The figure shows three views and two pictorial views of one solid part (mm, origin at its lowest corner). Answer the questions. Give positions to 0.01 mm unless a question says otherwise; leave off trailing zeros. Loops run counter-clockwise (first coordinate to the right, second up) from the corner with the lowest first, then second, coordinate; pieces in that order, holes last. Notation, with made-up numbers: (20, -30) - (77, -30) arc R37 ccw to (77, 7) - close; hole circle Ø5 at (26.5, 7.5). An arc over 180 degrees is marked (long way). One line per question, with ' | ' between items.
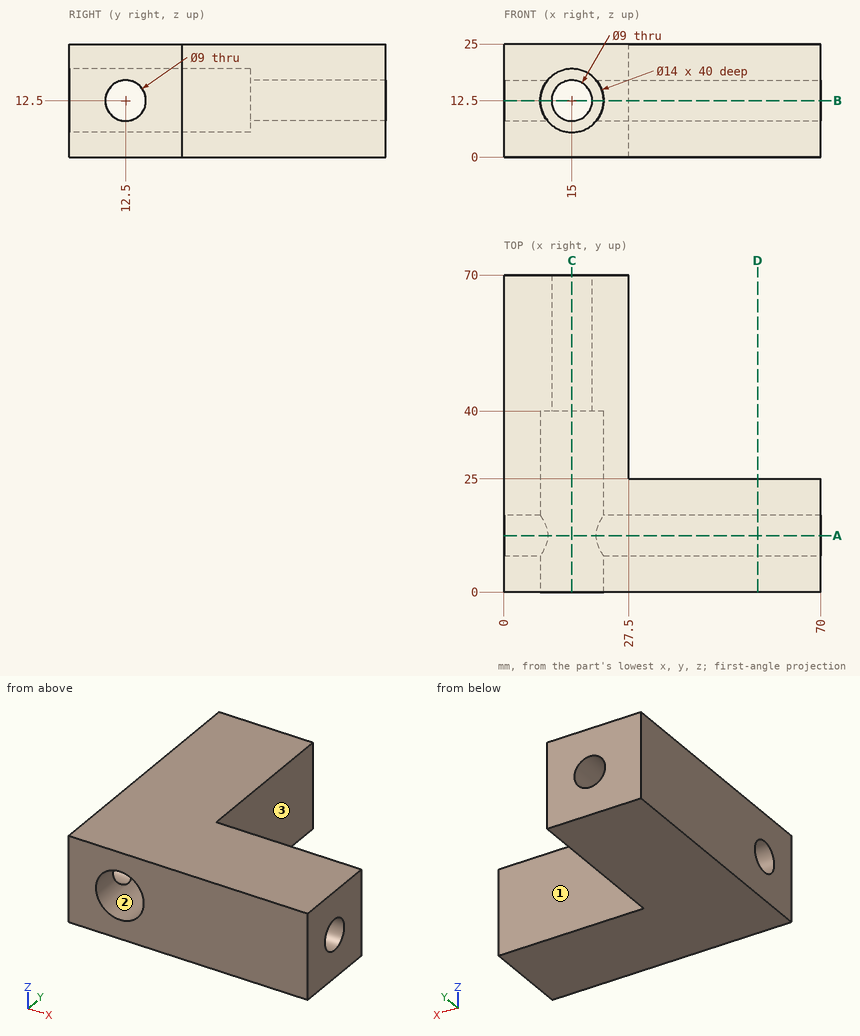
1. Find section B-B on z = 12.5. Write down the section's boundary in (x, y).
Evaluation:
outline: (0, 0) - (8, 0) - (8, 8) - (0, 8) - close; (0, 17) - (8, 17) - (8, 40) - (10.5, 40) - (10.5, 70) - (0, 70) - close; (19.5, 40) - (22, 40) - (22, 17) - (70, 17) - (70, 25) - (27.5, 25) - (27.5, 70) - (19.5, 70) - close; (22, 0) - (70, 0) - (70, 8) - (22, 8) - close
2. Find section D-D on x = 56. Write down the section's boundary in (y, z), then the cut area to 3 significant figures.
Evaluation:
outline: (0, 0) - (25, 0) - (25, 25) - (0, 25) - close; hole circle Ø9 at (12.5, 12.5) | area: 561 mm2
3. Consider L1, parallel to Z at x = 15, y = 48; L2, parallel to Y at x = 60, z = 12.25; L3, parallel to Y at x = 4, z = 12.5. Determine where each line is inside the solid, lowest interval first.
Evaluation:
L1: 0 to 8, 17 to 25 | L2: 0 to 8.01, 16.99 to 25 | L3: 0 to 8, 17 to 70
4. Determine the mould class of the marked faces 1, 2 and 3 for opening direction X: +X half, -X half, draft (parallel to the pull), parting line (faces both ways), or undercut.
Evaluation:
face 1: draft | face 2: undercut | face 3: +X half
5. Find section A-A on y = 12.5. Write down the section's boundary in (x, z).
Evaluation:
outline: (0, 0) - (70, 0) - (70, 8) - (20.36, 8) arc R7 cw to (9.64, 8) - (0, 8) - close; (0, 17) - (9.64, 17) arc R7 cw to (20.36, 17) - (70, 17) - (70, 25) - (0, 25) - close
6. Flat-ended cylindrical pins translate along their axes: pin 1 (2 mm diameter, centred on x = 13.5, z = 9, fed in from -Y); pin 2 (7.5 mm diameter, centred on x = 42, z = 11, fed in from +Y). Find the tip coordinate at first contact, or state that the pin passes through.
Evaluation:
pin 1: y = 40 | pin 2: y = 25
7. Find section C-C on x = 15. Write down the section's boundary in (y, z).
Evaluation:
outline: (0, 0) - (70, 0) - (70, 8) - (40, 8) - (40, 5.5) - (0, 5.5) - close; (0, 19.5) - (40, 19.5) - (40, 17) - (70, 17) - (70, 25) - (0, 25) - close
